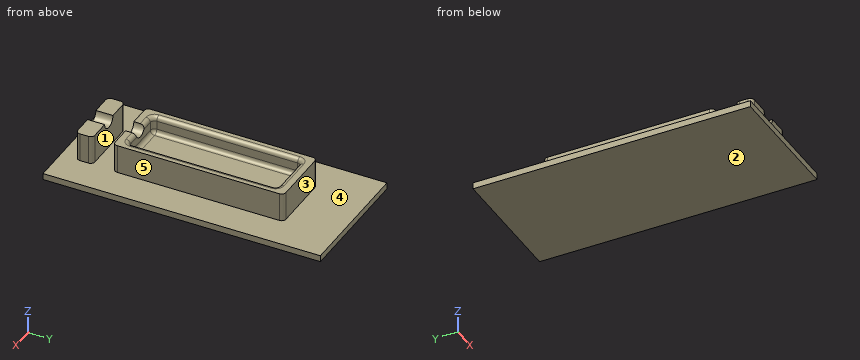
from build123d import *

# Parameters (mm, degrees)
F0_W      = 76.2
F0_H      = 203.2
F1_DEPTH  = 19.05
F2_W      = 55.88
F2_H      = 177.8
F3_DEPTH  = 20.32
F4_F1_R   = 5.08
F4_F2_R   = 5.08
F6_DEPTH  = 25.4
F7_W      = 152.4
F7_H      = 330.2
F7_W_2    = 76.2
F7_H_2    = 203.2
F8_DEPTH  = 3.81
F9_W      = 73.66
F9_H      = 20.32
F10_DEPTH = 34.29
F12_DEPTH = 25.4
F13_R     = 5.08


with BuildPart() as f1:
    # F0 (on Top) → F1 (new body, symmetric)
    with BuildSketch(Plane.XY):
        Rectangle(F0_W, F0_H)
    extrude(amount=F1_DEPTH, both=True)

    # F2 (on face) → F3 (cut)
    with BuildSketch(Plane.XY.offset(19.05)):
        Rectangle(F2_W, F2_H)
    extrude(amount=-F3_DEPTH, mode=Mode.SUBTRACT)

    # F4: fillet of radius 5.08 on 9 edges, made by hand

    # F4_f1
    f4_f1_edges = [f1.edges().sort_by_distance(p)[0] for p in [
        (-27.94, 0, -1.27),
        (0, 88.9, -1.27),
        (27.94, 0, -1.27),
        (0, -88.9, -1.27),
        (-27.94, 88.9, 8.89),
        (27.94, 88.9, 8.89),
        (27.94, -88.9, 8.89),
        (-27.94, -88.9, 8.89),
    ]]
    fillet(f4_f1_edges, radius=F4_F1_R)

    # F4_f2
    f4_f2_edges = [f1.edges().sort_by_distance(p)[0] for p in [
        (0, 88.9, 19.05),
        (26.4521024484, 87.4121024484, 19.05),
        (-26.4521024484, 87.4121024484, 19.05),
    ]]
    fillet(f4_f2_edges, radius=F4_F2_R)

    # F5 (on face) → F6 (cut)
    with BuildSketch(Plane.XZ.offset(101.6)):
        with BuildLine():
            Line((9.525, 19.05), (-9.525, 19.05))
            ThreePointArc((-9.525, 19.05), (0, 9.525), (9.525, 19.05))
        make_face()
    extrude(amount=-F6_DEPTH, mode=Mode.SUBTRACT)

    # F7 (on face) → F8 (join, symmetric)
    with BuildSketch(Plane(origin=(0, 0, -19.05), x_dir=(1, 0, 0), z_dir=(0, 0, -1))):
        Rectangle(F7_W, F7_H)
        Rectangle(F7_W_2, F7_H_2, mode=Mode.SUBTRACT)
        Rectangle(F7_W_2, F7_H_2)
    extrude(amount=F8_DEPTH, both=True)

    # F9 (on face) → F10 (join)
    with BuildSketch(Plane.XY.offset(-15.24)):
        with Locations((0, -136.5740124)):
            Rectangle(F9_W, F9_H)
    extrude(amount=F10_DEPTH)

    # F11 (on face) → F12 (cut)
    with BuildSketch(Plane.XZ.offset(146.7340124)):
        with BuildLine():
            Line((9.525, 19.05), (-9.525, 19.05))
            ThreePointArc((-9.525, 19.05), (0, 9.525), (9.525, 19.05))
        make_face()
    extrude(amount=-F12_DEPTH, mode=Mode.SUBTRACT)

    # F13
    f13_edges = [f1.edges().sort_by_distance(p)[0] for p in [
        (38.1, -101.6, 1.905),
        (36.83, -126.414012, 1.905),
        (36.83, -146.734012, 1.905),
        (-36.83, -146.734012, 1.905),
        (-36.83, -126.414012, 1.905),
        (-38.1, -101.6, 1.905),
        (38.1, 101.6, 1.905),
        (-38.1, 101.6, 1.905),
    ]]
    fillet(f13_edges, radius=F13_R)


solid = f1.part
Can you work these out from the model? Positions are in its coordinate system, mm. Face numbers are marked on the shaded views. A direction names the side the tool comes from. Round coordinates to 2 decimals unless told otherwise and drop trailing zeros. Loops run counter-clockwise (first coordinate to the right, second up) from the corner with the lowest first, then second, coordinate; pieces in that order, holes last. Notation, with made-up numbers: (70, 88) - (104, 88) arc R14 ccw to (104, 99) - close; hole circle Ø3 at (-4.75, -4). An arc over 180 degrees is marked (long way). Write item = value, one per line. Start each with the question number.
(1) For P1, Ø10.5, axis at x = -1, z = 3, coming from the -Y side; P2, Ø6, axis at y = 5.5, z = 12.5, coming from the -X side; P3, Ø17, axis at x = 7, z = 5.5, coming from the +Y side, each with a flat end and sliding along its axis, tell me the tip position at first contact or that it passes through.
(2) If I drill on probe 1 along Y at (x, z) = (-19.5, 5.5); probe 2 along Y at (x, z) = (31, 11); probe 3 along Y at (x, z) = (24.5, 2), over which ranges is the centre line in solid material (lowest first)? Write a range as [from, to].
(3) If we section it at A-A (x = 0): Please give me the cut outline in (y, z) (3 decimals), and give its area (3 significant figures).
(4) If we section it at C-C (x = -50): Please give me the cut outline in (y, z).
(5) If we section it at B-B (y = 24): Please give me the cut outline in (x, z).
(6) If we mould it in two halves opening along Y, with no side actions, what happens to the marked faces 1, 2 and 3? For each: released by +Y, released by -Y, zero draft, split by the parting line, or undercut.
(7) For the marked faces 4 and 5, which set-ups out of +Z, -Z, +X, -X, +Y, -Y let a thin tool reach every point of the face, with its end or its side?
Ans:
q1.P1 = -146.73
q1.P2 = -38.1
q1.P3 = 101.6
q2.probe_1 = [-146.73, -126.41], [-101.6, -88.9], [88.9, 101.6]
q2.probe_2 = [-146.73, -126.41], [-101.6, 101.6]
q2.probe_3 = [-146.73, -126.41], [-101.6, -88.27], [88.27, 101.6]
q3.outline = (-165.1, -22.86) - (165.1, -22.86) - (165.1, -15.24) - (101.6, -15.24) - (101.6, 19.05) - (93.98, 19.05) arc R5.08 ccw to (88.9, 13.97) - (88.9, 3.81) arc R5.08 cw to (83.82, -1.27) - (-83.82, -1.27) arc R5.08 cw to (-88.9, 3.81) - (-88.9, 9.525) - (-101.6, 9.525) - (-101.6, -15.24) - (-126.414, -15.24) - (-126.414, 9.525) - (-146.734, 9.525) - (-146.734, -15.24) - (-165.1, -15.24) - close
q3.area = 6,260 mm²
q4.outline = (-165.1, -22.86) - (165.1, -22.86) - (165.1, -15.24) - (-165.1, -15.24) - close
q5.outline = (-76.2, -22.86) - (76.2, -22.86) - (76.2, -15.24) - (38.1, -15.24) - (38.1, 19.05) - (33.02, 19.05) arc R5.08 ccw to (27.94, 13.97) - (27.94, 3.81) arc R5.08 cw to (22.86, -1.27) - (-22.86, -1.27) arc R5.08 cw to (-27.94, 3.81) - (-27.94, 13.97) arc R5.08 ccw to (-33.02, 19.05) - (-38.1, 19.05) - (-38.1, -15.24) - (-76.2, -15.24) - close
q6.face_1 = undercut
q6.face_2 = zero draft
q6.face_3 = released by +Y
q7.face_4 = +Z
q7.face_5 = +Z, +X, +Y, -Y
